```python
from build123d import *

# Parameters (mm, degrees)
SKETCH034_W             = 29.5
SKETCH034_H             = 13
PAD022_DEPTH            = 13.5
SKETCH035_R             = 1.75
PAD023_DEPTH            = 1.5
SKETCH036_W             = 10.1
SKETCH036_H             = 6.2
PAD024_DEPTH            = 8
BODY006_PLACEMENT_ANGLE = 180


with BuildPart() as part:
    # Sketch034 → Pad022 (new body)
    with BuildSketch(Plane.XZ):
        Rectangle(SKETCH034_W, SKETCH034_H)
    extrude(amount=PAD022_DEPTH)

    # Sketch035 (on Face5 of Pad022) → Pad023 (join)
    with BuildSketch(Plane(origin=(0, 0, 0), x_dir=(1, 0, 0), z_dir=(0, 1, 0))):
        with BuildLine():
            ThreePointArc((-18.7, 3.75), (-22.45, 0), (-18.7, -3.75))
            Line((18.69999, -3.75), (-18.7, -3.75))
            ThreePointArc((18.69999, -3.75), (22.45, -5e-06), (18.7, 3.75))
            Line((-18.7, 3.75), (18.7, 3.75))
        make_face()
        with Locations((-18.7, 0)):
            Circle(SKETCH035_R, mode=Mode.SUBTRACT)
        with Locations((18.7, 0)):
            Circle(SKETCH035_R, mode=Mode.SUBTRACT)
    extrude(amount=-PAD023_DEPTH)

    # Sketch036 (on Face10 of Pad023) → Pad024 (join)
    with BuildSketch(Plane(origin=(0, 0, -6.5), x_dir=(1, 0, 0), z_dir=(0, 0, -1))):
        with Locations((0, 6.8)):
            Rectangle(SKETCH036_W, SKETCH036_H)
    extrude(amount=PAD024_DEPTH)


with BuildPart() as part_1:
    # Body006 placement: moved
    add(part.part.moved(Location((-82.5, 61.5, 20))).rotate(Axis((-82.5, 61.5, 20), (0, 1, 0)), BODY006_PLACEMENT_ANGLE))


solid = part_1.part
```
Here's how the part is built. I have some questions about the finished solid (model axes, mm). A direction names the side the tool comes from. Coordinates: 2 decimals unless noted, no trailing zeros. Loops run counter-clockwise (first coordinate to the right, second up) from the corner with the lowest first, then second, coordinate; pieces in that order, holes last. Notation, with made-up numbers: (75.25, 42) - (125.25, 42) arc R28 ccw to (125.25, 69) - close; hole circle Ø11 at (-23.5, 22.5). An arc over 180 degrees is marked (long way). Return JSON: item names as keys, results as strings. Group by question number.
Item 1: On a 3-axis mill with a long thin cutter (end or side, diameter ignored), from which of +Z, -Z, +X, -X, +Y, -Y can I reach the whole of each face in a straight line? I mean faces 4 (the face through (-82, 57.8, 30)), 5 (the face through (-77.45, 55, 30)), 6 (the face through (-99, 61, 16.25)). Say none if no direction works.
Item 2: Will these pins go through, and if not, where does the flat tip stop? P1, Ø1.9, axis at y = 55, z = 31, coming from the -X side; P2, Ø1.2, axis at x = -66, y = 60.5, coming from the +Z side; P3, Ø4, axis at x = -83.5, z = 29, coming from the -Y side.
Item 3: If we section it at D-D on z = 24.75: Write out the boundary of the cut face in (x, y), and give its area (3 significant figures).
Item 4: If we section it at C-C on x = -79: Write out the boundary of the cut face in (y, z), and give its area (3 significant figures).
Item 5: We'd pull the mould along Z, two halves only. Please class faces 1 (the face through (-97.25, 55, 20)), 2 (the face through (-102.1, 60.8, 21.5)), 3 (the face through (-99, 61, 23.75)): +Z half, -Z half, draft (parallel to the pull), parting line (faces both ways), or undercut.
Item 6: I need wall thicknesses on line 1 (Z direction, x = -63.8, y = 61); line 2 (Y direction, x = -65.5, z = 18); line 3 (Z direction, x = -89, y = 60.5). Which ranges of each line are inside material? Lowest first, please. Write a range as from..to.
Item 7: If we section it at B-B on y = 53: Write out the boundary of the cut face in (x, z).
Item 8: If we section it at A-A on z = 20: Write out the boundary of the cut face in (x, y), and give its area (3 significant figures).
Calculated:
{
 "1": {"face 4": "+Z, +X, -X, +Y", "face 5": "+Z, +X, +Y, -Y", "face 6": "-Z, -X, +Y, -Y"},
 "2": {"P1": "stops at x = -87.55", "P2": "stops at z = 23.75", "P3": "stops at y = 51.6"},
 "3": {"outline": "(-97.25, 48) - (-67.75, 48) - (-67.75, 61.5) - (-97.25, 61.5) - close", "area": "398 mm^2"},
 "4": {"outline": "(48, 13.5) - (61.5, 13.5) - (61.5, 26.5) - (57.8, 26.5) - (57.8, 34.5) - (51.6, 34.5) - (51.6, 26.5) - (48, 26.5) - close", "area": "225 mm^2"},
 "5": {"face 1": "draft", "face 2": "undercut", "face 3": "+Z half"},
 "6": {"line 1": "z = 16.25..18.25, 21.75..23.75", "line 2": "y = 60..61.5", "line 3": "z = 13.5..26.5"},
 "7": {"outline": "(-97.25, 13.5) - (-67.75, 13.5) - (-67.75, 26.5) - (-77.45, 26.5) - (-77.45, 34.5) - (-87.55, 34.5) - (-87.55, 26.5) - (-97.25, 26.5) - close"},
 "8": {"outline": "(-104.95, 60) - (-102.95, 60) - (-102.95, 61.5) - (-104.95, 61.5) - close; (-99.45, 60) - (-97.25, 60) - (-97.25, 48) - (-67.75, 48) - (-67.75, 60) - (-65.55, 60) - (-65.55, 61.5) - (-99.45, 61.5) - close; (-62.05, 60) - (-60.05, 60) - (-60.05, 61.5) - (-62.05, 61.5) - close", "area": "411 mm^2"}
}
